Can you work these out from the model? Positions are in its coordinate system, mm. A direction names the side the tool comes from. Round coordinates to 2 decimals unless told otherwise and drop trailing zeros. Write each loop counter-clockwise with the first axis right and the second up, starting at its lowest first coordinate (ties: lowest second). Pieces come first, ordered by that corner, then holes. Notation, with made-up numbers: M -36,-36.75 L -15,-36.75 A29 cw -15,0.25 Z; hole C 60,-30 d2. An arc over 180 degrees is marked long. Answer in a Markdown table with one row per item. Add a question column.
(1) If we mould it in two halves opening along X, with no side actions, what happens to faces 3 (the face through (-15.861, 7.858, -7.745)), 4 (the face through (0, 5.5, 0)), 5 (the face through (15, 8, 0))? For each: released by +X, released by -X, zero draft, split by the parting line, or undercut.
(2) Suppose I cut it at A-A, the plane y = 10.75. Write out the boundary of the cut face in (x, z), then the cut area to 3 significant figures.
(3) Suppose I cut it at D-D, the plane x = -15. Write out the boundary of the cut face in (y, z), then the cut area to 4 significant figures.
(4) If I drill on probe 1 along X at (y, z) = (7.5, 2.75); probe 2 along X at (y, z) = (11.5, -7); probe 3 along Y at (x, z) = (1, -1), over which ranges is the centre line in solid material (lowest first)?
(5) I'm going to push flat-ended pins straight in: pin 1 (3 mm diameter, centred on x = 0, z = 2, fed in from +Y); pin 2 (1 mm diameter, centred on y = 8.5, z = -4.5, fed in from -X). Where does each tip first touch, or does it pass through?
(6) For faces 1 (the face through (-18, 8, 0)), 2 (the face through (3, 11, 0)), which set-ups out of +Z, -Z, +X, -X, +Y, -Y let a thin tool reach every point of the face, with its end or its side?
(7) Suppose I cut it at C-C, the plane z = -1.25. Write out the boundary of the cut face in (x, y), then the cut area to 4 significant figures.
(8) Suppose I cut it at B-B, the plane y = 2.5. Write out the boundary of the cut face in (x, z), then the cut area to 3 significant figures.
from build123d import *

# Parameters (mm, degrees)
CROQUIS1_W              = 33
CROQUIS1_H              = 20
SALIENTE_EXTRUIR1_DEPTH = 15.5
CROQUIS6_W              = 6
CROQUIS6_H              = 20
CORTAR_EXTRUIR2_DEPTH   = 10
REDONDEO1_R             = 7.5


with BuildPart() as part:
    # Croquis1 → Saliente-Extruir1 (new body)
    with BuildSketch(Plane(origin=(0, 0, 0), x_dir=(1, 0, 0), z_dir=(0, 1, 0))):
        with Locations((-1.5, 0)):
            Rectangle(CROQUIS1_W, CROQUIS1_H)
    extrude(amount=SALIENTE_EXTRUIR1_DEPTH)

    # Croquis6 → Cortar-Extruir2 (cut)
    with BuildSketch(Plane(origin=(0, 15.5, 0), x_dir=(1, 0, 0), z_dir=(0, 1, 0))):
        Rectangle(CROQUIS6_W, CROQUIS6_H)
    extrude(amount=-CORTAR_EXTRUIR2_DEPTH, mode=Mode.SUBTRACT)

    # Redondeo1
    redondeo1_edges = [part.edges().sort_by_distance(p)[0] for p in [
        (15, 7.75, 10),
        (-18, 7.75, 10),
        (-18, 7.75, -10),
        (15, 7.75, -10),
    ]]
    fillet(redondeo1_edges, radius=REDONDEO1_R)


solid = part.part
Calculated:
| question | item | result |
|---|---|---|
| 1 | face 3 | released by -X |
| 1 | face 4 | undercut |
| 1 | face 5 | released by +X |
| 2 | outline | M -18,-2.5 A7.5 ccw -10.5,-10 L -3,-10 L -3,10 L -10.5,10 A7.5 ccw -18,2.5 Z; M 3,-10 L 7.5,-10 A7.5 ccw 15,-2.5 L 15,2.5 A7.5 ccw 7.5,10 L 3,10 Z |
| 2 | area | 492 mm² |
| 3 | outline | M 0,-8.5 L 15.5,-8.5 L 15.5,8.5 L 0,8.5 Z |
| 3 | area | 263.5 mm² |
| 4 | probe 1 | -18 to -3, 3 to 15 |
| 4 | probe 2 | -16.5 to -3, 3 to 13.5 |
| 4 | probe 3 | 0 to 5.5 |
| 5 | pin 1 | y = 5.5 |
| 5 | pin 2 | x = -17.85 |
| 6 | face 1 | +Z, -Z, -X, +Y, -Y |
| 6 | face 2 | +Z, -Z, +Y |
| 7 | outline | M -18,0 L 15,0 L 15,15.5 L 3,15.5 L 3,5.5 L -3,5.5 L -3,15.5 L -18,15.5 Z |
| 7 | area | 451.5 mm² |
| 8 | outline | M -18,-2.5 A7.5 ccw -10.5,-10 L 7.5,-10 A7.5 ccw 15,-2.5 L 15,2.5 A7.5 ccw 7.5,10 L -10.5,10 A7.5 ccw -18,2.5 Z |
| 8 | area | 612 mm² |
